The listing builds one solid part. Answer for the finished solid, in the listing's coordinates (mm). A direction names the side the tool comes from. Round coordinates to 2 decimals unless told otherwise and drop trailing zeros. Order: outer loops, then holes, each group sorted by start corner. A loop starts at its lowest first (then second) coordinate and runs counter-clockwise, first axis right, second up. Notation, with made-up numbers: (28.25, -14.75) - (41.25, -14.75) arc R13 ccw to (41.25, -5.75) - close; hole circle Ø8 at (52.25, -9). An arc over 180 degrees is marked (long way). One line per item, written item: value. Start each with the question number.
1. For a pull along X with two mould halves and no side action, classify faces 3 (the flat face through (44, 0, 10)), 4 (the cylindrical face through (20.5, -0.5, 9.6)) as released by +X, released by -X, zero draft, split by the parting line, or undercut.
2. A flat-ended cylindrical pin translates along its axis: P1, Ø8, axis at x = 73, z = 11.5, coming from the -Y side. Find the tip coordinate at first contact, or state that the pin passes through.
3. Straight lines are drawn through the part: line 1 (X direction, y = -0.35, z = 9.5); line 2 (Z direction, x = 10, y = -0.75); line 3 (X direction, y = -0.5, z = 8.75). For each, find the intervals that lie inside material, in ascending order.
4. Section C-C, the plane z = 12 is taken. Give the vertices of the cut face in (x, y).
5. Section B-B, the plane x = 16 is taken. Give the vertices of the cut face in (y, z), then the cut area to 3 significant figures.
6. A tool of negligible diameter and unlimited length cuts with its end or side. For faces 1 (the cylindrical face through (3.5, -0.5, 9.4)), 2 (the flat face through (44, -1, 10)), from which of +Z, -Z, +X, -X, +Y, -Y can it reach the whole face along a straight path? Write none if from no direction.
7. Section A-A, the plane y = -0.75 is taken. Give the vertices of the cut face in (x, z), then the cut area to 3 significant figures.
from build123d import *

# Parameters (mm, degrees)
F0_W     = 90
F0_H     = 19
F1_DEPTH = 1
F2_SIZE  = 1
F3_SIZE  = 1
F4_SIZE  = 1
F5_SIZE  = 1


# Not quite as in the source:
# - ends of sketch curves that miss each other by under 0.0002 mm in the source are joined


with BuildPart() as f1:
    # F0 (on Front) → F1 (new body)
    with BuildSketch(Plane.XZ):
        with Locations((45, 9.5)):
            Rectangle(F0_W, F0_H)
        with BuildLine():
            Line((17, 6), (7, 6))
            ThreePointArc((7, 6), (3.5, 9.5), (7, 13))
            Line((7, 13), (17, 13))
            ThreePointArc((17, 13), (20.4999967813, 9.5), (17, 6))
        make_face(mode=Mode.SUBTRACT)
        with BuildLine():
            ThreePointArc((83, 13), (86.5, 9.5), (83, 6))
            Line((83, 6), (73.0000032187, 6))
            ThreePointArc((73.0000032187, 6), (69.5000032187, 9.5), (73.0000032187, 13))
            Line((73.0000032187, 13), (83, 13))
        make_face(mode=Mode.SUBTRACT)
    extrude(amount=F1_DEPTH)

    # F2
    f2_edges = [f1.edges().sort_by_distance(p)[0] for p in [
        (90, -0.5, 19),
    ]]
    chamfer(f2_edges, length=F2_SIZE)

    # F3
    f3_edges = [f1.edges().sort_by_distance(p)[0] for p in [
        (90, -0.5, 0),
    ]]
    chamfer(f3_edges, length=F3_SIZE)

    # F4
    f4_edges = [f1.edges().sort_by_distance(p)[0] for p in [
        (0, -0.5, 19),
    ]]
    chamfer(f4_edges, length=F4_SIZE)

    # F5
    f5_edges = [f1.edges().sort_by_distance(p)[0] for p in [
        (0, -0.5, 0),
    ]]
    chamfer(f5_edges, length=F5_SIZE)


solid = f1.part
Answer list:
1. face 3: zero draft
1. face 4: undercut
2. P1: stops at y = -1
3. line 1: x = 0 to 3.5, 20.5 to 69.5, 86.5 to 90
3. line 2: z = 0 to 6, 13 to 19
3. line 3: x = 0 to 3.58, 20.42 to 69.58, 86.42 to 90
4. outline: (0, -1) - (4.55, -1) - (4.55, 0) - (0, 0) - close; (19.45, -1) - (70.55, -1) - (70.55, 0) - (19.45, 0) - close; (85.45, -1) - (90, -1) - (90, 0) - (85.45, 0) - close
5. outline: (-1, 0) - (0, 0) - (0, 6) - (-1, 6) - close; (-1, 13) - (0, 13) - (0, 19) - (-1, 19) - close
5. area: 12.0 mm²
6. face 1: +Y, -Y
6. face 2: +Z, -Z, +X, -X, -Y
7. outline: (0, 1) - (1, 0) - (89, 0) - (90, 1) - (90, 18) - (89, 19) - (1, 19) - (0, 18) - close; hole (7, 6) - (17, 6) arc R3.5 ccw to (17, 13) - (7, 13) arc R3.5 ccw to start; hole (73, 6) - (83, 6) arc R3.5 ccw to (83, 13) - (73, 13) arc R3.5 ccw to start
7. area: 1,490 mm²
